Geometry check sheet. Reference: the model listing, model coordinates, mm. Face numbers are marked on the shaded views. Give positions to 0.01 mm unless a question says otherwise; leave off trailing zeros. Write each loop counter-clockwise with the first axis right and the second up, starting at its lowest first coordinate (ties: lowest second). Pieces come first, ordered by that corner, then holes.
(1) Thickness scan on line 1 along X through (y, z) = (128.5, -2) (1 decimal); line 2 along X through (y, z) = (149.5, -4); line 3 along X through (y, z) = (39, -0.25) (3 decimals). Record the ranges inside material, lowest first.
(2) Cross-section at A-A (y = 40). Record the boundary of the cut face in (x, z) (1 decimal).
(3) Depth check by flat-ended pin: P1, Ø3, axis at x = 97, y = 132.5, coming from the -Z side; P2, Ø4, axis at y = 96.5, z = -4.5, coming from the +X side; P3, Ø1, axis at y = 78, z = -5, coming from the +X side. Enter the tip coordinate at first touch or a pass-through.
(4) Mould release check, pull along Y, two halves, no side actions. Record for the marked faces 1 and 2: +Y half, -Y half, draft (parallel to the pull), parting line (faces both ways), or undercut.
(5) Cross-section at C-C (y = 138). Record the boundary of the cut face in (x, z) (1 decimal), and give its area (3 significant figures).
```python
from build123d import *

# Parameters (mm, degrees)
SKETCH3_W           = 117.475
SKETCH3_H           = 184.15
BOSS_EXTRUDE2_DEPTH = 3.175
FILLET1_R           = 3.81
SKETCH13_W          = 111.125
SKETCH13_H          = 177.8
SKETCH13_W_2        = 107.95
SKETCH13_H_2        = 174.625
BOSS_EXTRUDE4_DEPTH = 3.175
SKETCH14_W          = 6.35
SKETCH14_H          = 6.35
BOSS_EXTRUDE5_DEPTH = 6.35
FILLET9_R           = 0.381
SKETCH15_R          = 1.5875
CUT_EXTRUDE9_DEPTH  = 6.35
CUT_EXTRUDE10_START = -6.35
SKETCH16_R          = 1.5875
CUT_EXTRUDE10_DEPTH = 6.35
SKETCH17_W          = 1.5875
SKETCH17_H          = 57.15
BOSS_EXTRUDE6_DEPTH = 4.7625
SKETCH18_W          = 1.5875
SKETCH18_H          = 57.15
BOSS_EXTRUDE7_DEPTH = 4.7625


with BuildPart() as part:
    # Sketch3 → Boss-Extrude2 (new body)
    with BuildSketch(Plane.XY):
        with Locations((58.7375, 92.075)):
            Rectangle(SKETCH3_W, SKETCH3_H)
    extrude(amount=BOSS_EXTRUDE2_DEPTH)

    # Fillet1
    # the kernel refuses this fillet: 3.81 mm, written as the material it takes off along each edge
    with BuildSketch(Plane(origin=(126.866776656, 0, 3.175), x_dir=(0, 0, -1), z_dir=(-1, 0, 0)), Plane(origin=(-9.391776656, 184.15, 3.175), x_dir=(0, 0, -1), z_dir=(1, 0, 0))) as fillet1_piece_1:
        with BuildLine():
            CenterArc((3.81, -3.756710662), FILLET1_R, 99.594068227, 80.405931773)
            Line((0, -3.756710662), (-0.0762, -3.756710662))
            Line((-0.0762, -3.756710662), (-0.0762, 0))
            Line((-0.0762, 0), (0, 0.0762))
            ThreePointArc((0, 0.0762), (1.5875, 0.0762), (3.1623, 0.075134213))
            Line((3.1623, 0.075134213), (3.175, 0))
        make_face()
    extrude(amount=136.258553311, mode=Mode.SUBTRACT)
    with BuildSketch(Plane(origin=(117.475, 193.541776656, 3.175), x_dir=(0, 0, -1), z_dir=(0, -1, 0)), Plane(origin=(0, -9.391776656, 3.175), x_dir=(0, 0, -1), z_dir=(0, 1, 0))) as fillet1_piece_2:
        with BuildLine():
            CenterArc((3.81, -3.756710662), FILLET1_R, 99.594068227, 80.405931773)
            Line((0, -3.756710662), (-0.0762, -3.756710662))
            Line((-0.0762, -3.756710662), (-0.0762, 0))
            Line((-0.0762, 0), (0, 0.0762))
            ThreePointArc((0, 0.0762), (1.5875, 0.0762), (3.1623, 0.075134213))
            Line((3.1623, 0.075134213), (3.175, 0))
        make_face()
    extrude(amount=202.933553311, mode=Mode.SUBTRACT)

    # Sketch13 → Boss-Extrude4 (add)
    with BuildSketch(Plane(origin=(0, 0, 0), x_dir=(-1, 0, 0), z_dir=(0, 0, -1))):
        with Locations((-58.7375, 92.075)):
            Rectangle(SKETCH13_W, SKETCH13_H)
        with Locations((-58.7375, 92.075)):
            Rectangle(SKETCH13_W_2, SKETCH13_H_2, mode=Mode.SUBTRACT)
    extrude(amount=BOSS_EXTRUDE4_DEPTH)

    # Sketch14 → Boss-Extrude5 (add)
    with BuildSketch(Plane(origin=(0, 0, 0), x_dir=(-1, 0, 0), z_dir=(0, 0, -1))):
        with Locations((-111.125, 177.8)):
            Rectangle(SKETCH14_W, SKETCH14_H)
        with Locations((-6.35, 177.8)):
            Rectangle(SKETCH14_W, SKETCH14_H)
        with Locations((-111.125, 6.35)):
            Rectangle(SKETCH14_W, SKETCH14_H)
        with Locations((-6.35, 6.35)):
            Rectangle(SKETCH14_W, SKETCH14_H)
    extrude(amount=BOSS_EXTRUDE5_DEPTH)

    # Fillet9
    fillet9_edges = [part.edges().sort_by_distance(p)[0] for p in [
        (107.95, 7.14375, 0),
        (110.33125, 9.525, 0),
        (4.7625, 92.075, 0),
        (9.525, 4.7625, -1.5875),
        (4.7625, 9.525, -1.5875),
        (7.14375, 9.525, 0),
        (9.525, 7.14375, 0),
        (112.7125, 92.075, 0),
        (110.33125, 174.625, 0),
        (112.7125, 174.625, -1.5875),
        (107.95, 179.3875, -1.5875),
        (107.95, 177.00625, 0),
        (4.7625, 174.625, -1.5875),
        (58.7375, 179.3875, 0),
        (9.525, 179.3875, -1.5875),
        (9.525, 177.00625, 0),
        (7.14375, 174.625, 0),
        (58.7375, 4.7625, 0),
        (107.95, 4.7625, -1.5875),
        (112.7125, 9.525, -1.5875),
    ]]
    fillet(fillet9_edges, radius=FILLET9_R)

    # Sketch15 → Cut-Extrude9 (cut)
    with BuildSketch(Plane(origin=(114.3, 0, 0), x_dir=(0, 0, -1), z_dir=(1, 0, 0))):
        with Locations(Location((3.175, 6.35, 0), (0, 0, 90))):
            Circle(SKETCH15_R)
        with Locations(Location((3.175, 177.8, 0), (0, 0, 90))):
            Circle(SKETCH15_R)
    extrude(amount=-CUT_EXTRUDE9_DEPTH, mode=Mode.SUBTRACT)

    # Sketch16 → Cut-Extrude10 (cut)
    with BuildSketch(Plane.ZY.offset(-3.175).offset(CUT_EXTRUDE10_START)):
        with Locations(Location((-3.175, 177.8, 0), (0, 0, 90))):
            Circle(SKETCH16_R)
        with Locations(Location((-3.175, 6.35, 0), (0, 0, 90))):
            Circle(SKETCH16_R)
    extrude(amount=CUT_EXTRUDE10_DEPTH, mode=Mode.SUBTRACT)

    # Sketch17 → Boss-Extrude6 (add)
    with BuildSketch(Plane(origin=(0, 0, 0), x_dir=(-1, 0, 0), z_dir=(0, 0, -1))):
        with Locations((-102.52075, 149.225)):
            Rectangle(SKETCH17_W, SKETCH17_H)
        with Locations((-14.95425, 149.225)):
            Rectangle(SKETCH17_W, SKETCH17_H)
    extrude(amount=BOSS_EXTRUDE6_DEPTH)

    # Sketch18 → Boss-Extrude7 (add)
    with BuildSketch(Plane(origin=(0, 0, 0), x_dir=(-1, 0, 0), z_dir=(0, 0, -1))):
        with Locations((-102.52075, 91.821)):
            Rectangle(SKETCH18_W, SKETCH18_H)
        with Locations((-14.95425, 91.821)):
            Rectangle(SKETCH18_W, SKETCH18_H)
    extrude(amount=BOSS_EXTRUDE7_DEPTH)


solid = part.part
```
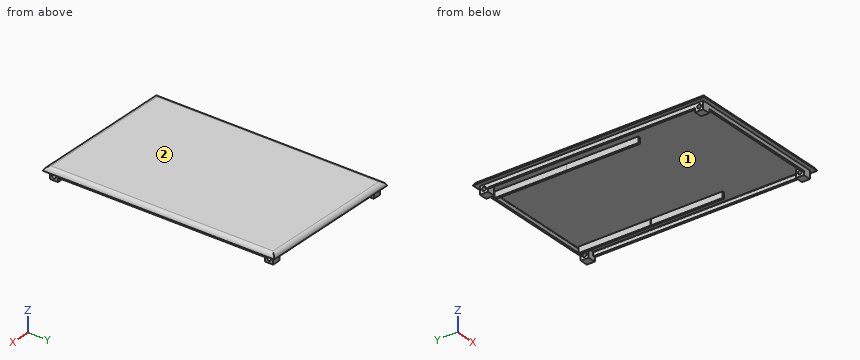
Reply:
1. line 1: x = 3.2 to 4.8, 14.2 to 15.7, 101.7 to 103.3, 112.7 to 114.3
1. line 2: x = 14.16 to 15.75, 101.73 to 103.31
1. line 3: x = 3.175 to 4.786, 112.689 to 114.3
2. outline: (0, 0) - (3.2, 0) - (3.2, -3.2) - (4.8, -3.2) - (4.8, -0.4) arc R0.4 cw to (5.1, 0) - (112.3, 0) arc R0.4 cw to (112.7, -0.4) - (112.7, -3.2) - (114.3, -3.2) - (114.3, 0) - (117.5, 0) arc R3.8 ccw to (113.7, 3.2) - (3.8, 3.2) arc R3.8 ccw to start
3. P1: stops at z = 0
3. P2: stops at x = 114.3
3. P3: stops at x = 103.31
4. face 1: undercut
4. face 2: draft
5. outline: (0, 0) - (3.2, 0) - (3.2, -3.2) - (4.8, -3.2) - (4.8, -0.4) arc R0.4 cw to (5.1, 0) - (14.2, 0) - (14.2, -4.8) - (15.7, -4.8) - (15.7, 0) - (101.7, 0) - (101.7, -4.8) - (103.3, -4.8) - (103.3, 0) - (112.3, 0) arc R0.4 cw to (112.7, -0.4) - (112.7, -3.2) - (114.3, -3.2) - (114.3, 0) - (117.5, 0) arc R3.8 ccw to (113.7, 3.2) - (3.8, 3.2) arc R3.8 ccw to start
5. area: 392 mm2
